Here's how the part is built. I have some questions about the finished solid (model axes, mm). Round coordinates to 2 decimals unless told otherwise and drop trailing zeros. Write each loop counter-clockwise with the first axis right and the second up, starting at its lowest first coordinate (ties: lowest second). Pieces come first, ordered by that corner, then holes. Notation, with made-up numbers: (26.25, -36.75) -> (47.25, -36.75) arc R16 ccw to (47.25, -26.75) -> close; hole circle Ø10 at (69.25, -39). An arc over 180 degrees is marked (long way). Put each result on its own line as item: value. Start each with the question number.
1) I want a section at C-C, the plane z = -154. List the corners of the cut face in (x, y) for me (3 decimals), then the cut area to 3 significant figures.
2) Will these pins go through, and if not, where does the flat tip stop? P1, Ø1.1, axis at x = 8.5, y = 1, coming from the -Z side (3 decimals); P2, Ø0.7, axis at x = 5.5, y = 1, coming from the +Z side (3 decimals).
3) I want a section at D-D, the plane x = 50.8. List the corners of the cut face in (y, z) for me (3 decimals).
4) I want a section at B-B, the plane y = 1.45. List the corners of the cut face in (x, z) for me (3 decimals).
5) We'd pull the mould along X, two halves only. Please class faces 1 (the cylindrical face through (206.073, 1.127, -237.547)), 2 (the flat face through (213, 2.286, -125)): released by +X, released by -X, zero draft, split by the parting line, or undercut.
6) I want a section at A-A, the plane x = 174. List the corners of the cut face in (y, z) for me, then the cut area to 3 significant figures.
7) If I drill on line 1 along Z through (x, y) = (203.2, 1.85) (3 decimals); line 2 along Z through (x, y) = (181.5, 0.9); line 3 along X through (y, z) = (1.4, -169.5) (3 decimals), over which ranges is the centre line in solid material (lowest first)? Write a range as [from, to].
Autodesk Inventor part; units mm, degrees
ref_plane "YZ Plane" through (0, 0, 0) normal (1, 0, 0) x (0, 1, 0)
ref_plane "XZ Plane" through (0, 0, 0) normal (0, 1, 0) x (-1, 0, 0)
ref_plane "XY Plane" through (0, 0, 0) normal (0, 0, 1) x (1, 0, 0)
sketch "Sketch1" plane through (0, 0, 0) normal (0, 1, 0) x (-1, 0, 0)
  line L0 (0, 0) -> (-254, 0)
  line L1 (-254, 0) -> (-254, -254)
  line L2 (-254, -254) -> (0, -254)
  line L3 (0, -254) -> (0, 0)
  line L4 (0, -15.875) -> (-10.287, -15.875)
  line L5 (-10.287, -15.875) -> (-10.287, 0)
  line L6 (-243.713, 0) -> (-243.713, -15.875)
  line L7 (-243.713, -15.875) -> (-254, -15.875)
  line L8 (-243.713, -254) -> (-243.713, -238.125)
  line L9 (-243.713, -238.125) -> (-254, -238.125)
  line L10 (-10.287, -254) -> (-10.287, -238.125)
  line L11 (-10.287, -238.125) -> (0, -238.125)
  dimension "d0" = 254
  dimension "d1" = 254
  dimension "d14" = 10.287
  dimension "d15" = 10.287
  dimension "d16" = 15.875
  dimension "d17" = 15.875
extrude "Extrusion1" add sketch "Sketch1" along normal blind 2.286 contours L5 L4 L3 L11 L10 L2 L8 L9 L1 L7 L6 L0
sketch "Sketch2" plane through (0, 2.286, 0) normal (0, 1, 0) x (1, 0, 0)
  line L0 (28.575, 31.75) -> (211.9884, 31.75)
  line L1 (211.9884, 31.75) -> (211.9884, 222.25)
  line L2 (211.9884, 222.25) -> (28.575, 222.25)
  line L3 (28.575, 222.25) -> (28.575, 31.75)
  line L4 (0, 15.875) -> (10.287, 15.875)
  line L5 (10.287, 15.875) -> (10.287, 0)
  line L6 (10.287, 0) -> (243.713, 0)
  line L7 (243.713, 0) -> (243.713, 15.875)
  line L8 (243.713, 15.875) -> (254, 15.875)
  line L9 (254, 15.875) -> (254, 238.125)
  line L10 (254, 238.125) -> (243.713, 238.125)
  line L11 (243.713, 238.125) -> (243.713, 254)
  line L12 (243.713, 254) -> (10.287, 254)
  line L13 (10.287, 254) -> (10.287, 238.125)
  line L14 (10.287, 238.125) -> (0, 238.125)
  line L15 (0, 238.125) -> (0, 15.875)
  line L16 (0, 238.125) -> (0, 15.875)
  point P0 (0, 0)
  point P1 (127, 0)
  point P2 (0, 127)
  point P3 (28.575, 127)
  point P4 (0, 127)
  dimension "d9" = 190.5
  dimension "d28" = 42.0116
  dimension "d29" = 28.575
extrude "Extrusion2" cut sketch "Sketch2" against normal through all contours L3 L2 L1 L0
sketch "Sketch3" plane through (0, 2.286, 0) normal (0, 1, 0) x (1, 0, 0)
  circle A0 centre (50.8, 9.525) radius 4
  circle A1 centre (203.2, 9.525) radius 4
  circle A2 centre (203.2, 244.475) radius 4.2037
  circle A3 centre (50.8, 244.475) radius 4.2037
  point P0 (0, 0)
hole "Hole1" at (50.8, 2.286, -9.525) at (50.8, 2.286, -244.475) at (203.2, 2.286, -244.475) at (203.2, 2.286, -9.525) direction (0, -1, 0) diameter 15 end through all
chamfer "Chamfer1" distance 3.175 angle 45 1 edges at (0, 1.143, -238.125)
equation "\"d15\" = d14"
equation "\"d17\" = d16"
properties part number "Carriage Sheet"
Findings:
1. outline: (0, 0) -> (28.575, 0) -> (28.575, 2.286) -> (0, 2.286) -> close; (211.988, 0) -> (254, 0) -> (254, 2.286) -> (211.988, 2.286) -> close
1. area: 161 mm2
2. P1: stops at z = -238.125
2. P2: stops at z = -15.875
3. outline: (0, -254) -> (2.286, -254) -> (2.286, -251.975) -> (0, -251.975) -> close; (0, -236.975) -> (2.286, -236.975) -> (2.286, -222.25) -> (0, -222.25) -> close; (0, -31.75) -> (2.286, -31.75) -> (2.286, -17.025) -> (0, -17.025) -> close; (0, -2.025) -> (2.286, -2.025) -> (2.286, 0) -> (0, 0) -> close
4. outline: (0, -234.95) -> (3.175, -238.125) -> (10.287, -238.125) -> (10.287, -254) -> (243.713, -254) -> (243.713, -238.125) -> (254, -238.125) -> (254, -15.875) -> (243.713, -15.875) -> (243.713, 0) -> (10.287, 0) -> (10.287, -15.875) -> (0, -15.875) -> close; hole (28.575, -222.25) -> (211.988, -222.25) -> (211.988, -31.75) -> (28.575, -31.75) -> close; hole circle Ø15 at (50.8, -244.475); hole circle Ø15 at (50.8, -9.525); hole circle Ø15 at (203.2, -244.475); hole circle Ø15 at (203.2, -9.525)
5. face 1: undercut
5. face 2: zero draft
6. outline: (0, -254) -> (2.29, -254) -> (2.29, -222.25) -> (0, -222.25) -> close; (0, -31.75) -> (2.29, -31.75) -> (2.29, 0) -> (0, 0) -> close
6. area: 145 mm2
7. line 1: z = [-254, -251.975], [-236.975, -222.25], [-31.75, -17.025], [-2.025, 0]
7. line 2: z = [-254, -222.25], [-31.75, 0]
7. line 3: x = [0, 28.575], [211.988, 254]
